```python
from build123d import *

# Parameters (mm, degrees)
F1_DEPTH       = 1050.925
F2_W           = 254
F2_H           = 273.05
F3_DEPTH       = 44.45
F5_D           = 26.9748
F5_CBORE_D     = 53.975
F5_CBORE_DEPTH = 3.175


with BuildPart() as f1:
    # F0 (on Right) → F1 (new body, symmetric)
    with BuildSketch(Plane.YZ):
        with BuildLine():
            Line((127, 126.746), (-127, 126.746))
            Line((-127, 126.746), (-127, 112.522))
            Line((-127, 112.522), (-22.098, 112.522))
            ThreePointArc((-22.098, 112.522), (-9.5256414305, 107.3143585695), (-4.318, 94.742))
            Line((-4.318, 94.742), (-4.318, -94.742))
            ThreePointArc((-4.318, -94.742), (-9.5256414305, -107.3143585695), (-22.098, -112.522))
            Line((-22.098, -112.522), (-127, -112.522))
            Line((-127, -112.522), (-127, -126.746))
            Line((-127, -126.746), (127, -126.746))
            Line((127, -126.746), (127, -112.522))
            Line((127, -112.522), (22.098, -112.522))
            ThreePointArc((22.098, -112.522), (9.5256414305, -107.3143585695), (4.318, -94.742))
            Line((4.318, -94.742), (4.318, 94.742))
            ThreePointArc((4.318, 94.742), (9.5256414305, 107.3143585695), (22.098, 112.522))
            Line((22.098, 112.522), (127, 112.522))
            Line((127, 112.522), (127, 126.746))
        make_face()
    extrude(amount=F1_DEPTH, both=True)

    # F2 (on face) → F3 (join)
    with BuildSketch(Plane.YZ.offset(1050.925)):
        Rectangle(F2_W, F2_H)
    extrude(amount=F3_DEPTH)

    # F5 (through all)
    with Locations(Plane(origin=(1050.925, 0, 0), x_dir=(0, -1, 0), z_dir=(-1, 0, 0))):
        with Locations((-88.9, 57.15), (-88.9, -57.15), (88.9, 57.15), (88.9, -57.15)):
            CounterBoreHole(F5_D / 2, F5_CBORE_D / 2, F5_CBORE_DEPTH)

    # F6: F1 across plane


with BuildPart() as f1_1:
    add(f1.part)
    add(f1.part.mirror(Plane.YZ))


solid = f1_1.part
```
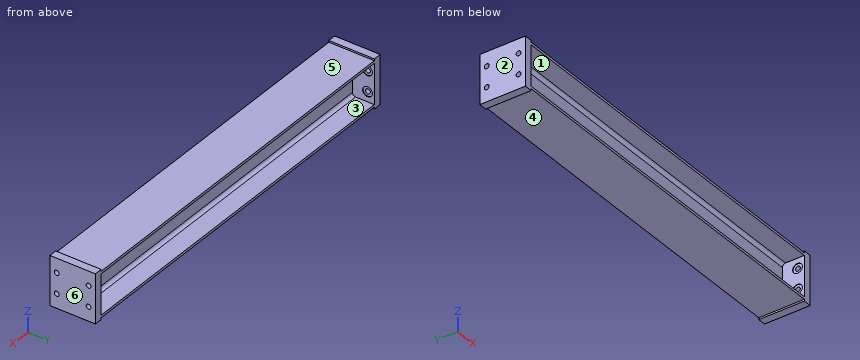
Could you check a few things on this model? Use its own coordinates, in mm. Face numbers are marked on the shaded views. A direction names the side the tool comes from. Round coordinates to 2 decimals unless told otherwise and drop trailing zeros. Write each loop counter-clockwise with the first axis right and the second up, starting at its lowest first coordinate (ties: lowest second). Pieces come first, ordered by that corner, then holes. Notation, with made-up numbers: M 83.25,12.5 L 112.25,12.5 A15 cw 112.25,27.5 Z; hole C 39.25,69.25 d11. An arc over 180 degrees is marked long. Write each question's results on one line, items separated by ' | '. Start each with the question number.
1. On a 3-axis mill with a long thin cutter (end or side, diameter ignored), from which of +Z, -Z, +X, -X, +Y, -Y can I reach the whole of each face in a straight line? I mean the marked faces 5 and 6. Say none if no direction works.
2. I'm going to push flat-ended pins straight in: pin 1 Ø6 at (x, z) = (149, 24) entering from +Y; pin 2 Ø8 at (x, z) = (356, -109) entering from -Y; pin 3 Ø5 at (x, y) = (-462.5, -45) entering from +Z; pin 4 Ø5 at (x, y) = (209, -47.5) entering from -Z. Where does each tip first touch, or does it pass through?
3. Imagine slicing it at A-A on x = 357.5. List the corners of the cut face in (y, z) for me, and give its area (3 significant figures).
4. I need wall thicknesses on L1, parallel to Y at x = 1072, z = 57; L2, parallel to Z at x = -1075.5, y = -88.9 (3 decimals); L3, parallel to Z at x = 1053.1, y = -88.9 (1 decimal). Which ranges of each line are inside material? Lowest first, please. Write a range as from..to.
5. Thinking about a two-plate mould opening in Z: for the marked faces 1, 2, 3 and 4, which applies, +Z half, -Z half, draft (parallel to the pull), parting line (faces both ways), or undercut?
Result sheet:
1) face 5: +Z, +Y, -Y | face 6: +Z, -Z, +X, +Y, -Y
2) pin 1: stops at y = 4.32 | pin 2: stops at y = -127 | pin 3: stops at z = 126.75 | pin 4: stops at z = -126.75
3) outline: M -127,-126.75 L 127,-126.75 L 127,-112.52 L 22.1,-112.52 A17.78 cw 4.32,-94.74 L 4.32,94.74 A17.78 cw 22.1,112.52 L 127,112.52 L 127,126.75 L -127,126.75 L -127,112.52 L -22.1,112.52 A17.78 cw -4.32,94.74 L -4.32,-94.74 A17.78 cw -22.1,-112.52 L -127,-112.52 Z | area: 9,440 mm^2
4) L1: y = -127..-102.39, -75.41..75.41, 102.39..127 | L2: z = -136.525..-70.637, -43.663..43.663, 70.637..136.525 | L3: z = -136.5..-84.1, -30.2..30.2, 84.1..136.5
5) face 1: undercut | face 2: draft | face 3: undercut | face 4: -Z half
